The listing builds one solid part. Answer for the finished solid, in the listing's coordinates (mm). A direction names the side the tool comes from. Give positions to 0.01 mm unless a question says otherwise; leave off trailing zeros. Write each loop counter-clockwise with the first axis right and the second up, starting at its lowest first coordinate (ties: lowest second). Pieces come first, ordered by that corner, then holes. Notation, with made-up numbers: M -7,-22.5 L 27,-22.5 A19 ccw 27,-5.5 Z; hole C 79,34.5 d6. An arc over 180 degrees is marked long. Answer as a JSON object with one key per item and string values.
```python
from build123d import *

# Parameters (mm, degrees)
F0_W     = 305
F0_H     = 95
F1_DEPTH = 10
F3_DEPTH = 25
F4_W     = 290
F4_H     = 5
F5_DEPTH = 3
F7_DEPTH = 25


with BuildPart() as f1:
    # F0 (on Right) → F1 (new body)
    with BuildSketch(Plane.YZ):
        with Locations((70.039693, 8.401494)):
            Rectangle(F0_W, F0_H)
    extrude(amount=F1_DEPTH)

    # F2 (on face) → F3 (cut)
    with BuildSketch(Plane.YZ.offset(10)):
        Polygon((-82.460307, 55.901494), (-82.460307, 40.901494), (-67.460307, 35.901494), (-67.460307, 55.901494), align=None)
        Polygon((-67.460307, 25.901494), (-82.460307, 20.901494), (-82.460307, -4.098506), (-67.460307, -9.098506), align=None)
        Polygon((-67.460307, -19.098506), (-82.460307, -24.098506), (-82.460307, -39.098506), (-67.460307, -39.098506), align=None)
    extrude(amount=-F3_DEPTH, mode=Mode.SUBTRACT)

    # F4 (on face) → F5 (cut)
    with BuildSketch(Plane(origin=(0, 0, 0), x_dir=(0, -1, 0), z_dir=(-1, 0, 0))):
        with Locations((-77.539693, -31.598506)):
            Rectangle(F4_W, F4_H)
    extrude(amount=-F5_DEPTH, mode=Mode.SUBTRACT)

    # F6 (on face) → F7 (cut)
    with BuildSketch(Plane.YZ.offset(10)):
        Polygon((212.539693, 35.901494), (222.539693, 40.901494), (222.539693, 55.901494), (212.539693, 55.901494), align=None)
        Polygon((222.539693, -4.098506), (222.539693, 20.901494), (212.539693, 25.901494), (212.539693, -9.098506), align=None)
        Polygon((222.539693, -39.098506), (222.539693, -24.098506), (212.539693, -19.098506), (212.539693, -39.098506), align=None)
    extrude(amount=-F7_DEPTH, mode=Mode.SUBTRACT)


solid = f1.part
```
1. For faces 1 (the flat face through (5.07, 217.47, 38.366)), 2 (the flat face through (5, 212.54, 9)), 3 (the flat face through (3, 74, -32)), determine the directions among +Z, -Z, +X, -X, +Y, -Y from which every point of the face is accessible in a straight line to the end or side of a thin tool.
Verdict:
{"face 1": "+Z, +X, -X", "face 2": "+X, -X", "face 3": "-X, +Y, -Y"}
2. The mould has two halves that part along Z. Classify faces 4 (the flat face through (5, -82.46, 31)), 5 (the flat face through (5.07, -75.07, -6.56)), 6 (the flat face through (5.07, -75.07, 38.44)): released by +Z, released by -Z, zero draft, split by the parting line, or undercut.
Verdict:
{"face 4": "zero draft", "face 5": "undercut", "face 6": "released by +Z"}
3. Consider line 1 along Z through (x, y) = (1.75, -21.5); line 2 along Y through (x, z) = (1.5, 48); line 3 along Z through (x, y) = (5.25, -68). Determine where each line is inside the solid, lowest interval first.
Verdict:
{"line 1": "z = -39.1 to -34.1, -29.1 to 55.9", "line 2": "y = -67.46 to 212.54", "line 3": "z = -19.28 to -8.92, 25.72 to 36.08"}
4. A cutting plane is placed at C-C, the plane z = 47.5. Give the vertices of the cut face in (x, y), plus the area to 3 significant figures.
Verdict:
{"outline": "M 0,-67.46 L 10,-67.46 L 10,212.54 L 0,212.54 Z", "area": "2,800 mm2"}
5. Flat-ended cylindrical pins translate along their axes: pin 1 (5.5 mm diameter, centred on y = 62, z = -30.5, fed in from -X); pin 2 (5 mm diameter, centred on x = 3, z = 5, fed in from -Y). Find the tip coordinate at first contact, or state that the pin passes through.
Verdict:
{"pin 1": "stops at x = 0", "pin 2": "stops at y = -67.46"}
6. A cutting plane is placed at B-B, the plane y = 161. Give the vertices of the cut face in (x, z), plus the area to 3 significant figures.
Verdict:
{"outline": "M 0,-39.1 L 10,-39.1 L 10,55.9 L 0,55.9 L 0,-29.1 L 3,-29.1 L 3,-34.1 L 0,-34.1 Z", "area": "935 mm2"}
7. A cutting plane is placed at A-A, the plane x = 7. Give the vertices of the cut face in (y, z), plus the area to 4 significant figures.
Verdict:
{"outline": "M -82.46,-24.1 L -67.46,-19.1 L -67.46,-39.1 L 212.54,-39.1 L 212.54,-19.1 L 222.54,-24.1 L 222.54,-4.1 L 212.54,-9.1 L 212.54,25.9 L 222.54,20.9 L 222.54,40.9 L 212.54,35.9 L 212.54,55.9 L -67.46,55.9 L -67.46,35.9 L -82.46,40.9 L -82.46,20.9 L -67.46,25.9 L -67.46,-9.1 L -82.46,-4.1 Z", "area": "27,350 mm2"}
